Read the model definition and answer for the solid it produces. Units are mm, in the model's axes. Face numbers are marked on the shaded views. A direction names the side the tool comes from. Coordinates: 2 decimals unless noted, no trailing zeros. Order: outer loops, then holes, each group sorted by start corner. A loop starts at its lowest first (then second) coordinate and runs counter-clockwise, first axis right, second up.
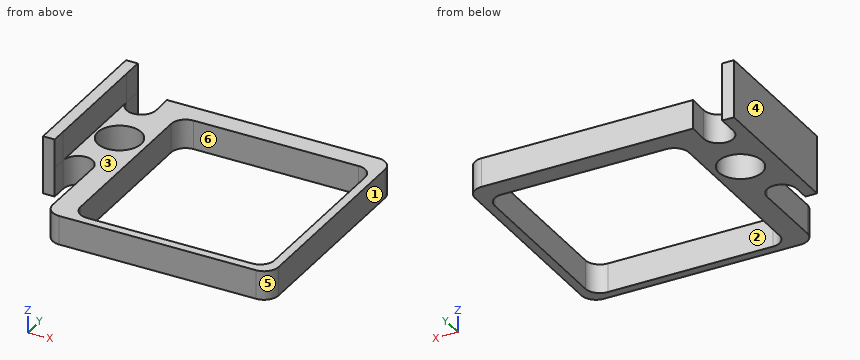
```python
from build123d import *

# Parameters (mm, degrees)
F1_DEPTH = 10
F3_DEPTH = 10
F2_R     = 7.5
F4_DEPTH = 25


# Not quite as in the source:
# - a feature names something its author has since deleted; it is built from what else it names


with BuildPart() as f1:
    # F0 (on Top) → F1 (new body)
    with BuildSketch(Plane.XY):
        with BuildLine():
            Line((-12.3976909148, -50), (55.6003173012, -50))
            ThreePointArc((55.6003173012, -50), (59.1358512071, -48.5355339059), (60.6003173012, -45))
            Line((60.6003173012, -45), (60.6003173012, 22))
            ThreePointArc((60.6003173012, 22), (59.1358512071, 25.5355339059), (55.6003173012, 27))
            Line((55.6003173012, 27), (-17.4436509052, 27))
            Line((-17.4436509052, 27), (-17.3007774584, 20.1056662166))
            ThreePointArc((-17.3007774584, 20.1056662166), (-22.3084516237, 14.9008160564), (-27.4991044794, 19.9232047976))
            Line((-27.4991044794, 19.9232047976), (-27.4991044794, 27))
            Line((-27.4991044794, 27), (-31.5450169146, 27))
            Line((-31.5450169146, 27), (-31.5450169146, -25.2973511815))
            Line((-31.5450169146, -25.2973511815), (-27.499666141, -25.2973511815))
            Line((-27.499666141, -25.2973511815), (-27.499666141, -19.9870042568))
            ThreePointArc((-27.499666141, -19.9870042568), (-22.3611815213, -14.9001453296), (-17.3000843541, -20.0640056487))
            Line((-17.3000843541, -20.0640056487), (-17.3976909148, -45))
            ThreePointArc((-17.3976909148, -45), (-15.9332248208, -48.5355339059), (-12.3976909148, -50))
        make_face()
        with BuildLine():
            ThreePointArc((52.6003173012, 20), (56.1358512071, 18.5355339059), (57.6003173012, 15))
            Line((57.6003173012, 15), (57.6003173012, -42))
            ThreePointArc((57.6003173012, -42), (56.1358512071, -45.5355339059), (52.6003173012, -47))
            Line((52.6003173012, -47), (-4.3996826988, -47))
            ThreePointArc((-4.3996826988, -47), (-7.9352166047, -45.5355339059), (-9.3996826988, -42))
            Line((-9.3996826988, -42), (-9.3996826988, 15))
            ThreePointArc((-9.3996826988, 15), (-7.9352166047, 18.5355339059), (-4.3996826988, 20))
            Line((-4.3996826988, 20), (52.6003173012, 20))
        make_face(mode=Mode.SUBTRACT)
    extrude(amount=F1_DEPTH)

    # F2 (on face) → F3 (join)
    with BuildSketch(Plane.XY.offset(10)):
        Polygon((-27.4991044794, 27), (-31.5450169146, 27), (-31.5450169146, -25.2973511815), (-27.499666141, -25.2973511815), (-27.4996091091, -19.9870042574), (-27.4991804826, 19.9232047984), align=None)
    extrude(amount=F3_DEPTH)

    # F2 (on face) → F4 (cut)
    with BuildSketch(Plane.XY.offset(10)):
        with Locations((-19, 0)):
            Circle(F2_R)
    extrude(amount=-F4_DEPTH, mode=Mode.SUBTRACT)


solid = f1.part
```
1) Straight lines are drawn through the part: line 1 (Y direction, x = 42.5, z = 9.75); line 2 (X direction, y = 10.5, z = 2.5); line 3 (Z direction, x = -12, y = -21.5). For each, find the intervals that lie inside material, in ascending order.
A:
line 1: y = -50 to -47, 20 to 27
line 2: x = -31.55 to -9.4, 57.6 to 60.6
line 3: z = 0 to 10
2) A cutting plane is placed at D-D, the plane y = -44. Determine the outline of the cut face in (x, z).
A:
outline: (-17.39, 0) - (-8.98, 0) - (-8.98, 10) - (-17.39, 10) - close; (57.18, 0) - (60.6, 0) - (60.6, 10) - (57.18, 10) - close
3) Which of the six approach directions +Z, -Z, +X, -X, +Y, -Y give full straight-line access (tool end or side, diameter ignored) to the marked faces 1, 2 and 3?
A:
face 1: +Z, -Z, +X, +Y, -Y
face 2: +Z, -Z
face 3: +Z, +X, +Y, -Y
4) A cutting plane is placed at C-C, the plane z = 7.5. Determine the outline of the cut face in (x, y).
A:
outline: (-31.55, -25.3) - (-27.5, -25.3) - (-27.5, -19.99) arc R5.1 cw (long way) to (-17.3, -20.06) - (-17.4, -45) arc R5 ccw to (-12.4, -50) - (55.6, -50) arc R5 ccw to (60.6, -45) - (60.6, 22) arc R5 ccw to (55.6, 27) - (-17.44, 27) - (-17.3, 20.11) arc R5.1 cw (long way) to (-27.5, 19.92) - (-27.5, 27) - (-31.55, 27) - close; hole circle Ø15 at (-19, 0); hole (-9.4, -42) arc R5 ccw to (-4.4, -47) - (52.6, -47) arc R5 ccw to (57.6, -42) - (57.6, 15) arc R5 ccw to (52.6, 20) - (-4.4, 20) arc R5 ccw to (-9.4, 15) - close
5) Determine the mould class of the marked faces 4, 5 and 6 for opening direction X: pulls with the +X half, pulls with the -X half, needs draft (parallel to the pull), parting line crosses it, or undercut.
A:
face 4: pulls with the -X half
face 5: pulls with the +X half
face 6: undercut
6) A cutting plane is placed at B-B, the plane y = -6. Determine the outline of the cut face in (x, z), and give its area (3 significant figures).
A:
outline: (-31.55, 0) - (-23.5, 0) - (-23.5, 10) - (-27.5, 10) - (-27.5, 20) - (-31.55, 20) - close; (-14.5, 0) - (-9.4, 0) - (-9.4, 10) - (-14.5, 10) - close; (57.6, 0) - (60.6, 0) - (60.6, 10) - (57.6, 10) - close
area: 202 mm2
7) Flat-ended cylindrical pins translate along their axes: pin 1 Ø8 at (y, z) = (24, 14.5) entering from +X; pin 2 Ø1.2 at (x, z) = (-30, 7) entering from -Y. Find the tip coordinate at first contact, or state that the pin passes through.
A:
pin 1: stops at x = -27.5
pin 2: stops at y = -25.3
8) A cutting plane is placed at A-A, the plane x = 54. Determine the outline of the cut face in (y, z).
A:
outline: (-50, 0) - (-46.8, 0) - (-46.8, 10) - (-50, 10) - close; (19.8, 0) - (27, 0) - (27, 10) - (19.8, 10) - close
